from build123d import *

# Parameters (mm, degrees)
CROQUIS1_R              = 2.35
SALIENTE_EXTRUIR1_DEPTH = 4
SALIENTE_EXTRUIR2_START = -4
CROQUIS2_W              = 10
CROQUIS2_H              = 6
SALIENTE_EXTRUIR2_DEPTH = 4
CORTAR_EXTRUIR1_DEPTH   = 0.1


with BuildPart() as part:
    # Croquis1 → Saliente-Extruir1 (new body, symmetric)
    with BuildSketch(Plane(origin=(0, 0, 0), x_dir=(1, 0, 0), z_dir=(0, 1, 0))):
        with BuildLine():
            Line((-8, 12), (8, 12))
            ThreePointArc((8, 12), (10.828427125, 10.828427125), (12, 8))
            Line((12, 8), (12, -8))
            ThreePointArc((12, -8), (10.828427125, -10.828427125), (8, -12))
            Line((8, -12), (-8, -12))
            ThreePointArc((-8, -12), (-10.828427125, -10.828427125), (-12, -8))
            Line((-12, -8), (-12, 8))
            ThreePointArc((-12, 8), (-10.828427125, 10.828427125), (-8, 12))
        make_face()
        with Locations((-8, 0)):
            Circle(CROQUIS1_R, mode=Mode.SUBTRACT)
        with Locations((8, 0)):
            Circle(CROQUIS1_R, mode=Mode.SUBTRACT)
    extrude(amount=SALIENTE_EXTRUIR1_DEPTH, both=True)

    # Croquis2 → Saliente-Extruir2 (add)
    with BuildSketch(Plane(origin=(0, 0, 0), x_dir=(1, 0, 0), z_dir=(0, 1, 0)).offset(SALIENTE_EXTRUIR2_START)):
        with Locations((0, -12)):
            Rectangle(CROQUIS2_W, CROQUIS2_H)
    extrude(amount=SALIENTE_EXTRUIR2_DEPTH)

    # Croquis3 → Cortar-Extruir1 (cut)
    with BuildSketch(Plane(origin=(0, 4, 0), x_dir=(1, 0, 0), z_dir=(0, 1, 0))):
        with BuildLine():
            Line((-8, 3), (-16.530379626, 3))
            Line((-16.530379626, 3), (-16.530379626, -3))
            Line((-16.530379626, -3), (-8, -3))
            ThreePointArc((-8, -3), (-5, 0), (-8, 3))
        make_face()
        with BuildLine():
            Line((16.530379626, -3), (8, -3))
            ThreePointArc((8, -3), (5, 0), (8, 3))
            Line((8, 3), (16.530379626, 3))
            Line((16.530379626, 3), (16.530379626, -3))
        make_face()
    cortar_extruir1 = extrude(amount=-CORTAR_EXTRUIR1_DEPTH, mode=Mode.SUBTRACT)

    # Simetría1: Cortar-Extruir1 across plane
    add(cortar_extruir1.mirror(Plane.ZX), mode=Mode.SUBTRACT)


solid = part.part
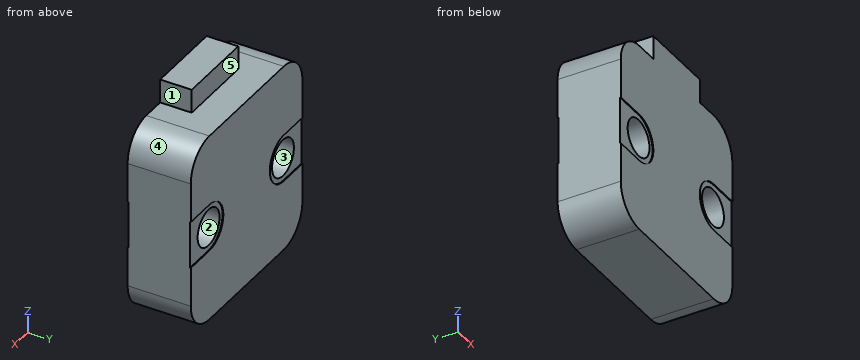
Source: CAD feature listing. Evaluate the final solid. Frame: model axes, mm. Face numbers are marked on the shaded views. A direction names the side the tool comes from. Coordinates: 2 decimals unless noted, no trailing zeros. Loops run counter-clockwise (first coordinate to the right, second up) from the corner with the lowest first, then second, coordinate; pieces in that order, holes last. Notation, with made-up numbers: (26, -8) - (52, -8) arc R26 ccw to (52, 22) - close; hole circle Ø6 at (69, 69). An arc over 180 degrees is marked (long way). Return JSON: item names as keys, results as strings.
Q1. Section D-D, the plane x = 2.75. Return loops of the section in (y, z).
Results:
{"outline": "(-4, -12) - (4, -12) - (4, 12) - (0, 12) - (0, 15) - (-4, 15) - close"}
Q2. Section B-B, the plane z = 0. Return loops of the section in (x, y), plus the area to 3 significant figures.
Results:
{"outline": "(-12, -3.9) - (-10.35, -3.9) - (-10.35, 3.9) - (-12, 3.9) - close; (-5.65, -3.9) - (-5, -3.9) - (-5, -4) - (5, -4) - (5, -3.9) - (5.65, -3.9) - (5.65, 3.9) - (5, 3.9) - (5, 4) - (-5, 4) - (-5, 3.9) - (-5.65, 3.9) - close; (10.35, -3.9) - (12, -3.9) - (12, 3.9) - (10.35, 3.9) - close", "area": "116 mm2"}
Q3. Material intervals for line 1 along X through (y, z) = (3.5, 0.5); line 2 along Z through (x, y) = (-8, 2.25); line 3 along X through (y, z) = (-3.25, 0.75), sorted ascending.
Results:
{"line 1": "-12 to -10.3, -5.7 to 5.7, 10.3 to 12", "line 2": "-12 to -2.35, 2.35 to 12", "line 3": "-12 to -10.23, -5.77 to 5.77, 10.23 to 12"}
Q4. Contact query for flat-ended pins moving along their axis: P1, Ø2.5, axis at y = -2, z = 14, coming from the -X side; P2, Ø2.5, axis at y = -2.5, z = 13.5, coming from the +X side. Output: stop coordinate, or through.
Results:
{"P1": "x = -5", "P2": "x = 5"}
Q5. Mould query, pull axis Z, two halves, no side actions, for the marked faces 3, 4 and 5. Classes: released by +Z, released by -Z, zero draft, split by the parting line, or undercut.
Results:
{"face 3": "undercut", "face 4": "released by +Z", "face 5": "zero draft"}
Q6. Section A-A, the plane y = 0.5. Return loops of the section in (x, z), plus the area to 3 significant figures.
Results:
{"outline": "(-12, -8) arc R4 ccw to (-8, -12) - (8, -12) arc R4 ccw to (12, -8) - (12, 8) arc R4 ccw to (8, 12) - (-8, 12) arc R4 ccw to (-12, 8) - close; hole circle Ø4.7 at (-8, 0); hole circle Ø4.7 at (8, 0)", "area": "528 mm2"}
Q7. Section C-C, the plane x = 9.75. Return loops of the section in (y, z), plus the area to 3 significant figures.
Results:
{"outline": "(-4, -11.6) - (4, -11.6) - (4, -3) - (3.9, -3) - (3.9, -1.57) - (-3.9, -1.57) - (-3.9, -3) - (-4, -3) - close; (-4, 3) - (-3.9, 3) - (-3.9, 1.57) - (3.9, 1.57) - (3.9, 3) - (4, 3) - (4, 11.6) - (-4, 11.6) - close", "area": "160 mm2"}
Q8. Access query for the marked faces 1 and 2. Directions: +Z, -Z, +X, -X, +Y, -Y. A direction counts if a zero-diameter tool reaches every point of the face in a straight line with its end or side. Return the directions, or none.
Results:
{"face 1": "+Z, +X, +Y, -Y", "face 2": "+Y, -Y"}
